Work out the finished part from the listing and answer in its coordinate system (mm). Face numbers are marked on the shaded views. A direction names the side the tool comes from. Round coordinates to 2 decimals unless told otherwise and drop trailing zeros. Order: outer loops, then holes, each group sorted by start corner. A loop starts at its lowest first (then second) coordinate and runs counter-clockwise, first axis right, second up. Notation, with made-up numbers: M 45,4 L 86,4 A6 ccw 86,14 Z; hole C -32.75,63.5 d11. An arc over 180 degrees is marked long. Return JSON: item names as keys, results as strings.
from build123d import *

# Parameters (mm, degrees)
SALIENTE_EXTRUIR1_DEPTH = 40
CROQUIS3_R              = 2.5
CORTAR_EXTRUIR1_DEPTH   = 94
CROQUIS5_W              = 40
CROQUIS5_H              = 10
CORTAR_EXTRUIR2_DEPTH   = 40
CROQUIS6_W              = 42
CROQUIS6_H              = 22
CORTAR_EXTRUIR3_DEPTH   = 10
CROQUIS7_R              = 2
CORTAR_EXTRUIR4_DEPTH   = 10
CROQUIS8_W              = 60
CROQUIS8_H              = 33
CROQUIS8_R              = 2
CROQUIS8_W_2            = 42
CROQUIS8_H_2            = 22
SALIENTE_EXTRUIR2_DEPTH = 4
CROQUIS9_W              = 99.924242424
CROQUIS9_H              = 56.811688312
CORTAR_EXTRUIR9_DEPTH   = 41


with BuildPart() as part:
    # Croquis2 → Saliente-Extruir1 (new body)
    with BuildSketch(Plane.XY):
        Polygon((-31.145916957, -11.001243781), (-31.145916957, 23.998756219), (53.854083043, 23.998756219), (53.854083043, -11.001243781), (57.854083043, -11.001243781), (57.854083043, 27.998756219), (-35.145916957, 27.998756219), (-35.145916957, -11.001243781), align=None)
    extrude(amount=SALIENTE_EXTRUIR1_DEPTH)

    # Croquis3 → Cortar-Extruir1 (cut, through all)
    with BuildSketch(Plane.ZY.offset(35.145916957)):
        with Locations((20, 7.998756219)):
            Circle(CROQUIS3_R)
    extrude(amount=-CORTAR_EXTRUIR1_DEPTH, mode=Mode.SUBTRACT)

    # Croquis5 → Cortar-Extruir2 (cut)
    with BuildSketch(Plane.ZY.offset(35.145916957)):
        with Locations((20, -6.001243781)):
            Rectangle(CROQUIS5_W, CROQUIS5_H)
    extrude(amount=-CORTAR_EXTRUIR2_DEPTH, mode=Mode.SUBTRACT)

    # Croquis6 → Cortar-Extruir3 (cut)
    with BuildSketch(Plane(origin=(0, 27.998756219, 0), x_dir=(1, 0, 0), z_dir=(0, 1, 0))):
        with Locations((11.354083043, -20)):
            Rectangle(CROQUIS6_W, CROQUIS6_H)
    extrude(amount=-CORTAR_EXTRUIR3_DEPTH, mode=Mode.SUBTRACT)

    # Croquis7 → Cortar-Extruir4 (cut)
    with BuildSketch(Plane(origin=(0, 27.998756219, 0), x_dir=(1, 0, 0), z_dir=(0, 1, 0))):
        with Locations((-13.645916957, -15)):
            Circle(CROQUIS7_R)
        with Locations((-13.645916957, -25)):
            Circle(CROQUIS7_R)
        with Locations((36.354083043, -15)):
            Circle(CROQUIS7_R)
        with Locations((36.354083043, -25)):
            Circle(CROQUIS7_R)
    extrude(amount=-CORTAR_EXTRUIR4_DEPTH, mode=Mode.SUBTRACT)

    # Croquis8 → Saliente-Extruir2 (add)
    with BuildSketch(Plane(origin=(0, 27.998756219, 0), x_dir=(1, 0, 0), z_dir=(0, 1, 0))):
        with Locations((11.354083043, -20)):
            Rectangle(CROQUIS8_W, CROQUIS8_H)
        with Locations((-8.895916957, -6.25)):
            Circle(CROQUIS8_R, mode=Mode.SUBTRACT)
        with Locations((1.104083043, -6.25)):
            Circle(CROQUIS8_R, mode=Mode.SUBTRACT)
        with Locations((-8.895916957, -33.75)):
            Circle(CROQUIS8_R, mode=Mode.SUBTRACT)
        with Locations((1.104083043, -33.75)):
            Circle(CROQUIS8_R, mode=Mode.SUBTRACT)
        with Locations((-13.645916957, -15)):
            Circle(CROQUIS8_R, mode=Mode.SUBTRACT)
        with Locations((-13.645916957, -25)):
            Circle(CROQUIS8_R, mode=Mode.SUBTRACT)
        with Locations((36.354083043, -15)):
            Circle(CROQUIS8_R, mode=Mode.SUBTRACT)
        with Locations((36.354083043, -25)):
            Circle(CROQUIS8_R, mode=Mode.SUBTRACT)
        with Locations((11.354083043, -20)):
            Rectangle(CROQUIS8_W_2, CROQUIS8_H_2, mode=Mode.SUBTRACT)
    extrude(amount=SALIENTE_EXTRUIR2_DEPTH)

    # Croquis9 → Cortar-Extruir9 (cut, through all)
    with BuildSketch(Plane.XY.offset(40)):
        with Locations((14.816204255, -0.407087937)):
            Rectangle(CROQUIS9_W, CROQUIS9_H)
    extrude(amount=-CORTAR_EXTRUIR9_DEPTH, mode=Mode.SUBTRACT)


solid = part.part
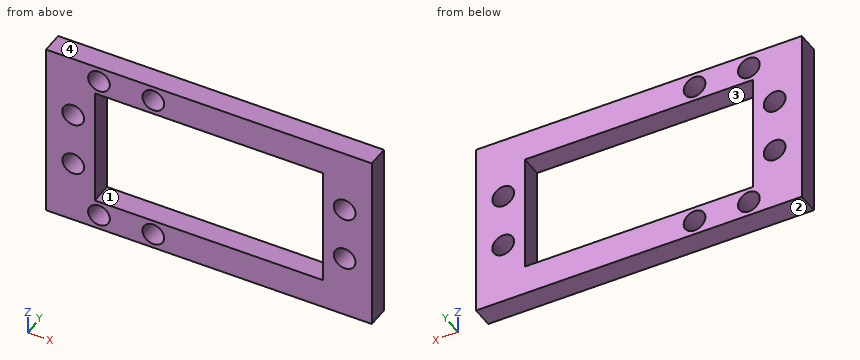
Item 1: Which of the six approach directions +Z, -Z, +X, -X, +Y, -Y give full straight-line access (tool end or side, diameter ignored) to the marked faces 1 and 2?
Output:
{"face 1": "+Y, -Y", "face 2": "-Z, +X, -X, +Y, -Y"}
Item 2: Find section B-B (x = 5). Determine the outline of the cut face in (y, z).
Output:
{"outline": "M 28,3.5 L 32,3.5 L 32,9 L 28,9 Z; M 28,31 L 32,31 L 32,36.5 L 28,36.5 Z"}
Item 3: Consider line 1 along X through (y, z) = (31, 15); line 2 along X through (y, z) = (28.8, 33.75); line 3 along Z through (x, y) = (-13.5, 29.8). Determine where each line is inside the solid, lowest interval first. Write a range as [from, to].
Output:
{"line 1": "x = [-18.65, -15.65], [-11.65, -9.65], [32.35, 34.35], [38.35, 41.35]", "line 2": "x = [-18.65, -10.9], [-6.9, -0.9], [3.1, 41.35]", "line 3": "z = [3.5, 13.01], [16.99, 23.01], [26.99, 36.5]"}
Item 4: Find section D-D (y = 30.85). State how many separate pieces and enclosed holes the cut face has, plus the area to 3 significant figures.
Output:
{"separate pieces": "1", "enclosed holes": "9", "area": "955 mm^2"}
Item 5: The mould has two halves that part along X. Classify the marked faces 3 and 4: pulls with the +X half, pulls with the -X half, needs draft (parallel to the pull), parting line crosses it, or undercut.
Output:
{"face 3": "undercut", "face 4": "needs draft"}
Item 6: Find section C-C (z = 6.25). Determine the outline of the cut face in (x, y).
Output:
{"outline": "M -18.65,28 L -10.9,28 L -10.9,32 L -18.65,32 Z; M -6.9,28 L -0.9,28 L -0.9,32 L -6.9,32 Z; M 3.1,28 L 41.35,28 L 41.35,32 L 3.1,32 Z"}
Item 7: Find section A-A (z = 15). Determine the outline of the cut face in (x, y), plus the area to 3 significant figures.
Output:
{"outline": "M -18.65,28 L -15.65,28 L -15.65,32 L -18.65,32 Z; M -11.65,28 L -9.65,28 L -9.65,32 L -11.65,32 Z; M 32.35,28 L 34.35,28 L 34.35,32 L 32.35,32 Z; M 38.35,28 L 41.35,28 L 41.35,32 L 38.35,32 Z", "area": "40.0 mm^2"}
